```python
from build123d import *

# Parameters (mm, degrees)
F0_W     = 25.4
F0_H     = 25.4
F1_DEPTH = 3.175
F3_W     = 5.08
F3_H     = 12.7
F6_DEPTH = 6.35
F7_R     = 4.572
F8_R     = 0.762


with BuildPart() as f1:
    # F0 (on Top) → F1 (new body)
    with BuildSketch(Plane.XY):
        Rectangle(F0_W, F0_H)
    extrude(amount=F1_DEPTH)

    # F4: sweep along a path in F2
    with BuildLine(Plane.XZ) as f4_path:
        ThreePointArc((-10.16, 0), (0, -23.55829), (10.16, 0))
    # F3 (on face) → F4 (sweep)
    with BuildSketch(Plane(origin=(0, 0, 0), x_dir=(1, 0, 0), z_dir=(0, 0, -1))):
        with Locations((-10.16, 0)):
            Rectangle(F3_W, F3_H)
    sweep(path=f4_path.line)

    # F5 (on Front) → F6 (join, symmetric)
    with BuildSketch(Plane.XZ):
        with BuildLine():
            Line((10.013058, -2.535746), (10.16, 0))
            Line((10.16, 0), (7.62, 0))
            ThreePointArc((7.62, 0), (8.907227, -1.182279), (10.013058, -2.535746))
        make_face()
    extrude(amount=F6_DEPTH, both=True)

    # F7
    f7_edges = [f1.edges().sort_by_distance(p)[0] for p in [
        (12.7, -12.7, 1.5875),
        (12.7, 12.7, 1.5875),
        (-12.7, 12.7, 1.5875),
        (-12.7, -12.7, 1.5875),
    ]]
    fillet(f7_edges, radius=F7_R)

    # F8
    f8_edges = [f1.edges().sort_by_distance(p)[0] for p in [
        (0, -12.7, 3.175),
        (-11.360892, -11.360892, 3.175),
        (11.360892, -11.360892, 3.175),
        (-12.7, 0, 3.175),
        (12.7, 0, 3.175),
        (-11.360892, 11.360892, 3.175),
        (11.360892, 11.360892, 3.175),
        (0, 12.7, 3.175),
    ]]
    fillet(f8_edges, radius=F8_R)


solid = f1.part
```
Geometry: final body of the model. Coordinates: model frame, mm. A direction names the side the tool comes from. Give positions to 0.01 mm unless a question says otherwise; leave off trailing zeros. Loops run counter-clockwise (first coordinate to the right, second up) from the corner with the lowest first, then second, coordinate; pieces in that order, holes last. Notation, with made-up numbers: (11.5, 35.25) -> (66.5, 35.25) arc R20 cw to (66.5, 65.25) -> close; hole circle Ø4 at (4, 82). An arc over 180 degrees is marked (long way). Use CSV: the item, a comma, the result in double quotes.
(1) First-contact query: P1, Ø4, axis at x = 2.5, y = -2, coming from the -Z side; P2, Ø1.2, axis at y = 0.5, z = 1, coming from the +X side; P3, Ø4, axis at x = -7.5, y = -7.5, coming from the -Z side; P4, Ø8, axis at y = -6.5, z = -10.5, coming from the +X side. Flat tips, straight axial feed; report the tip coordinate or a pass-through.
From the geometry:
P1,"z = -25.49"
P2,"x = 12.7"
P3,"z = -24.38"
P4,"x = 15.91"
(2) Cut plane C-C (z = -7.5). Output: boundary loops of the cut face in (x, y).
From the geometry:
outline,"(-15.78, -6.35) -> (-12.07, -6.35) -> (-12.07, 6.35) -> (-15.78, 6.35) -> close; (12.07, -6.35) -> (15.78, -6.35) -> (15.78, 6.35) -> (12.07, 6.35) -> close"
(3) Cut plane A-A (x = 0). Output: boundary loops of the cut face in (y, z) (3 decimals).
From the geometry:
outline,"(-12.7, 0) -> (12.7, 0) -> (12.7, 2.413) arc R0.762 ccw to (11.938, 3.175) -> (-11.938, 3.175) arc R0.762 ccw to (-12.7, 2.413) -> close; (-6.35, -25.501) -> (6.35, -25.501) -> (6.35, -21.836) -> (-6.35, -21.836) -> close"
(4) Access query for faces 4 (the face through (-12.7, 0, 1)), 5 (the face through (0, -6.35, -22)), 6 (the face through (8.89, -0.089, -1.164)), 7 (the face through (12.7, 0, 1)), 8 (the face through (0, 6.35, -22)). Directions: +Z, -Z, +X, -X, +Y, -Y. A direction counts if a zero-diameter tool reaches every point of the face in a straight line with its end or side. Return the directions, or none.
From the geometry:
face 4,"+Z, -X, +Y, -Y"
face 5,"-Z, +X, -X, -Y"
face 6,"+Y, -Y"
face 7,"+Z, +X, +Y, -Y"
face 8,"-Z, +X, -X, +Y"
(5) Pull-direction query (Z, two-part tool) for faces 1 (the face through (0, 0, 3.175)), 2 (the face through (-11.325, -11.396, 1.223)), 3 (the face through (0, 0, 0)); classes: released by +Z, released by -Z, zero draft, split by the parting line, or undercut.
From the geometry:
face 1,"released by +Z"
face 2,"zero draft"
face 3,"undercut"
(6) Cut plane B-B (y = 4.75). Output: boundary loops of the cut face in (x, z) (3 decimals).
From the geometry:
outline,"(-12.7, 0) arc R15.913 ccw (long way) to (12.7, 0) -> (12.7, 2.413) arc R0.762 ccw to (11.938, 3.175) -> (-11.938, 3.175) arc R0.762 ccw to (-12.7, 2.413) -> close; hole (-7.62, 0) arc R12.247 ccw (long way) to (10.013, -2.536) arc R12.247 ccw to (7.62, 0) -> close"
(7) Ray query, line 1 along Z through (x, y) = (0, 3.5) (3 decimals); line 2 along Y through (x, z) = (-10, -19.5); line 3 along X through (y, z) = (-6.25, -17.5). Return the intervals inside material, ascending. Write a range as [from, to].
From the geometry:
line 1,"[-25.501, -21.836], [0, 3.175]"
line 2,"[-6.35, 6.35]"
line 3,"[-13.81, -9.35], [9.35, 13.81]"
